```python
from build123d import *

# Parameters (mm, degrees)
SKETCH1_R           = 15
BOSS_EXTRUDE1_DEPTH = 2
SKETCH2_W           = 15
SKETCH2_H           = 6
BOSS_EXTRUDE2_DEPTH = 25
SKETCH3_W           = 15
SKETCH3_H           = 20
BOSS_EXTRUDE3_DEPTH = 5
CHAMFER1_SIZE       = 4
SKETCH4_R           = 1
CUT_EXTRUDE1_DEPTH  = 15


with BuildPart() as part:
    # Sketch1 → Boss-Extrude1 (new body)
    with BuildSketch(Plane(origin=(0, 0, 0), x_dir=(1, 0, 0), z_dir=(0, 1, 0))):
        with Locations(Location((0, 0, 0), (0, 0, 270))):
            Circle(SKETCH1_R)
    extrude(amount=BOSS_EXTRUDE1_DEPTH)

    # Sketch2 → Boss-Extrude2 (add)
    with BuildSketch(Plane(origin=(0, 2, 0), x_dir=(1, 0, 0), z_dir=(0, 1, 0))):
        Rectangle(SKETCH2_W, SKETCH2_H)
    extrude(amount=BOSS_EXTRUDE2_DEPTH)

    # Sketch3 → Boss-Extrude3 (add)
    with BuildSketch(Plane(origin=(0, 27, 0), x_dir=(1, 0, 0), z_dir=(0, 1, 0))):
        with Locations((0, -7)):
            Rectangle(SKETCH3_W, SKETCH3_H)
    extrude(amount=BOSS_EXTRUDE3_DEPTH)

    # Chamfer1
    chamfer1_edges = [part.edges().sort_by_distance(p)[0] for p in [
        (0, 27, 3),
    ]]
    chamfer(chamfer1_edges, length=CHAMFER1_SIZE)

    # Sketch4 → Cut-Extrude1 (cut)
    with BuildSketch(Plane(origin=(7.5, 0, 0), x_dir=(0, 0, -1), z_dir=(1, 0, 0))):
        with Locations((-14, 29.5)):
            Circle(SKETCH4_R)
    extrude(amount=-CUT_EXTRUDE1_DEPTH, mode=Mode.SUBTRACT)


solid = part.part
```
Design review of the part built by this model. Coordinates are the model's own, in mm. A direction names the side the tool comes from. Give positions to 0.01 mm unless a question says otherwise; leave off trailing zeros. Write each loop counter-clockwise with the first axis right and the second up, starting at its lowest first coordinate (ties: lowest second). Pieces come first, ordered by that corner, then holes. Notation, with made-up numbers: (32.25, 48.5) - (36.25, 48.5) arc R7 cw to (36.25, 61.5) - close; hole circle Ø2 at (85.5, -20.5). An arc over 180 degrees is marked (long way). Return JSON: item names as keys, results as strings. Group by question number.
(1) We need section C-C, the plane z = 8. Give the boundary of the cut face in (x, y), then the cut area to 3 significant figures.
(2) Insertion check: pin 1 (7.5 mm diameter, centred on x = -1, y = 17.5, fed in from +Z); pin 2 (1.8 mm diameter, centred on y = 29.5, z = 14, fed in from -X); pin 3 (1.5 mm diameter, centred on x = -5.5, z = -10.5, fed in from +Y); pin 4 (1 mm diameter, centred on y = 28, z = 7, fed in from +X). Each pin has a flat end and moves straight along its axis. Give the tip position at first contact, or say it passes through.
(3) To check wall thickness, follow probe 1 along Y at (x, z) = (4.25, 14); probe 2 along Z at (x, y) = (2, 13.5); probe 3 along Y at (x, z) = (-7.75, 9). State the ranges of each line that lie inside material, in increasing order.
(4) We need section B-B, the plane x = 0. Give the boundary of the cut face in (y, z), then the cut area to 3 significant figures.
(5) Machinability: for faces 4 (the flat face through (0, 12, 3)), 5 (the flat face through (0, 17, -3)), 6 (the flat face through (7.5, 20.1, 2.7)), which of the approach directions +Z, -Z, +X, -X, +Y, -Y give a long, thin tool a straight path to every point of the face, cutting with its end or side? Answer none if there is none.
(6) We need section D-D, the plane z = 0. Give the boundary of the cut face in (x, y), then the cut area to 3 significant figures.
(7) Mouldability with a two-part tool opening along Z and no side actions: class faces 1 (the flat face through (0, 29, 17)), 2 (the flat face through (0, 2, -4)), 3 (the cylindrical face through (0.11, 30.34, 13.46)) as +Z half, -Z half, draft (parallel to the pull), parting line (faces both ways), or undercut.
(8) We need section A-A, the plane y = 29.5. Give the boundary of the cut face in (x, z).
Reported:
{
 "1": {"outline": "(-12.69, 0) - (12.69, 0) - (12.69, 2) - (-12.69, 2) - close; (-7.5, 27) - (7.5, 27) - (7.5, 32) - (-7.5, 32) - close", "area": "126 mm2"},
 "2": {"pin 1": "stops at z = 3", "pin 2": "passes through", "pin 3": "stops at y = 2", "pin 4": "stops at x = 7.5"},
 "3": {"probe 1": "y = 0 to 2, 27 to 28.5, 30.5 to 32", "probe 2": "z = -3 to 3", "probe 3": "y = 0 to 2"},
 "4": {"outline": "(0, -15) - (2, -15) - (2, -3) - (32, -3) - (32, 17) - (27, 17) - (27, 7) - (23, 3) - (2, 3) - (2, 15) - (0, 15) - close; hole circle Ø2 at (29.5, 14)", "area": "315 mm2"},
 "5": {"face 4": "+Z, +X, -X", "face 5": "-Z, +X, -X, +Y", "face 6": "+Z, -Z, +X, +Y"},
 "6": {"outline": "(-15, 0) - (15, 0) - (15, 2) - (7.5, 2) - (7.5, 32) - (-7.5, 32) - (-7.5, 2) - (-15, 2) - close", "area": "510 mm2"},
 "7": {"face 1": "+Z half", "face 2": "draft", "face 3": "undercut"},
 "8": {"outline": "(-7.5, -3) - (7.5, -3) - (7.5, 13) - (-7.5, 13) - close; (-7.5, 15) - (7.5, 15) - (7.5, 17) - (-7.5, 17) - close"}
}
